Here's how the part is built. I have some questions about the finished solid (model axes, mm). A direction names the side the tool comes from. Coordinates: 2 decimals unless noted, no trailing zeros. Write each loop counter-clockwise with the first axis right and the second up, starting at its lowest first coordinate (ties: lowest second). Pieces come first, ordered by that corner, then holes.
(1) Thinking about a two-plate mould opening in X: for faces 6 (the flat face through (0, -25.5, 0)), 7 (the flat face through (0, -33.1, 0)), 8 (the cylindrical face through (37.46, -15.53, 0.99)), 9 (the flat face through (-36, -12, 0)), which applies, released by +X, released by -X, zero draft, split by the parting line, or undercut?
(2) Please list where these lines run through material, in increasing order: probe 1 along Y at (x, z) = (0, 1.15); probe 2 along X at (y, z) = (0, 2.45); probe 3 along X at (y, z) = (-32, 1).
(3) Imagine slicing it at B-B, the plane x = 0. List the corners of the cut face in (y, z) for me, plus the area to 3 significant figures.
(4) For pin 1 Ø10 at (x, y) = (30.5, -15.5) entering from -Z; pin 2 Ø1 at (x, z) = (-4.5, -1.5) entering from -Y; pin 3 Ø4 at (y, z) = (-30, 0) entering from -X, each with a flat end and sliding along its axis, tell me the tip position at first contact or that it passes through.
(5) Imagine slicing it at A-A, the plane y = 0. List the corners of the cut face in (x, z) for me.
(6) Which directions (+Z, -Z, +X, -X, +Y, -Y) give clear straight access to the entire face, cutting with the end or side of a thin tool? Please do faces 1 (the cylindrical face through (-0.1, -37.5, -2)), 2 (the flat face through (-10, -31, 0)), 3 (the flat face through (7.5, -31, 0)), 4 (the flat face through (33, -21, 1.4)), 5 (the flat face through (0, -34, -4)).
```python
from build123d import *

# Parameters (mm, degrees)
F0_R     = 40.55
F0_W     = 15
F0_H     = 5.2
F1_DEPTH = 1.4
F2_DEPTH = 3.4
F3_DEPTH = 4
F4_R     = 0.6
F5_R     = 2
F6_R     = 0.6


with BuildPart() as f1:
    # F0 (on Top) → F1 (new body)
    with BuildSketch(Plane.XY):
        Circle(F0_R)
        with BuildLine():
            ThreePointArc((-10, -37.4374478297), (-23.6015094856, 30.7332271329), (38.75, 0))
            ThreePointArc((38.75, 0), (30.7332271329, -23.6015094856), (10, -37.4374478297))
            Line((10, -37.4374478297), (10, -39))
            Line((10, -39), (-10, -39))
            Line((-10, -39), (-10, -37.4374478297))
        make_face(mode=Mode.SUBTRACT)
        with BuildLine():
            ThreePointArc((10, -37.4374478297), (30.7332271329, -23.6015094856), (38.75, 0))
            ThreePointArc((38.75, 0), (-23.6015094856, 30.7332271329), (-10, -37.4374478297))
            Line((-10, -37.4374478297), (-10, -36.142080737))
            ThreePointArc((-10, -36.142080737), (-22.7073776557, 29.8433409658), (37.5, 0))
            ThreePointArc((37.5, 0), (29.8433409658, -22.7073776557), (10, -36.142080737))
            Line((10, -36.142080737), (10, -37.4374478297))
        make_face()
        with BuildLine():
            Line((-10, -25.5), (-10, -36.142080737))
            ThreePointArc((-10, -36.142080737), (0, -37.5), (10, -36.142080737))
            Line((10, -36.142080737), (10, -25.5))
            Line((10, -25.5), (-10, -25.5))
        make_face()
        with Locations((0, -30.5)):
            Rectangle(F0_W, F0_H, mode=Mode.SUBTRACT)
        with BuildLine():
            Line((-10, -36.142080737), (-10, -37.4374478297))
            ThreePointArc((-10, -37.4374478297), (0, -38.75), (10, -37.4374478297))
            Line((10, -37.4374478297), (10, -36.142080737))
            ThreePointArc((10, -36.142080737), (0, -37.5), (-10, -36.142080737))
        make_face()
        with BuildLine():
            ThreePointArc((10, -37.4374478297), (0, -38.75), (-10, -37.4374478297))
            Line((-10, -37.4374478297), (-10, -39))
            Line((-10, -39), (10, -39))
            Line((10, -39), (10, -37.4374478297))
        make_face()
    extrude(amount=F1_DEPTH)

    # F0 (on Top) → F2 (join)
    with BuildSketch(Plane.XY):
        with BuildLine():
            ThreePointArc((10, -37.4374478297), (30.7332271329, -23.6015094856), (38.75, 0))
            ThreePointArc((38.75, 0), (-23.6015094856, 30.7332271329), (-10, -37.4374478297))
            Line((-10, -37.4374478297), (-10, -36.142080737))
            ThreePointArc((-10, -36.142080737), (-22.7073776557, 29.8433409658), (37.5, 0))
            ThreePointArc((37.5, 0), (29.8433409658, -22.7073776557), (10, -36.142080737))
            Line((10, -36.142080737), (10, -37.4374478297))
        make_face()
        with BuildLine():
            Line((-10, -36.142080737), (-10, -37.4374478297))
            ThreePointArc((-10, -37.4374478297), (0, -38.75), (10, -37.4374478297))
            Line((10, -37.4374478297), (10, -36.142080737))
            ThreePointArc((10, -36.142080737), (0, -37.5), (-10, -36.142080737))
        make_face()
        with BuildLine():
            Line((-10, -25.5), (-10, -36.142080737))
            ThreePointArc((-10, -36.142080737), (0, -37.5), (10, -36.142080737))
            Line((10, -36.142080737), (10, -25.5))
            Line((10, -25.5), (-10, -25.5))
        make_face()
        with Locations((0, -30.5)):
            Rectangle(F0_W, F0_H, mode=Mode.SUBTRACT)
    extrude(amount=F2_DEPTH)

    # F0 (on Top) → F3 (join)
    with BuildSketch(Plane.XY):
        with BuildLine():
            Line((-10, -25.5), (-10, -36.142080737))
            ThreePointArc((-10, -36.142080737), (0, -37.5), (10, -36.142080737))
            Line((10, -36.142080737), (10, -25.5))
            Line((10, -25.5), (-10, -25.5))
        make_face()
        with Locations((0, -30.5)):
            Rectangle(F0_W, F0_H, mode=Mode.SUBTRACT)
    extrude(amount=-F3_DEPTH)

    # F4
    f4_edges = [f1.edges().sort_by_distance(p)[0] for p in [
        (-40.55, 0, 0),
    ]]
    fillet(f4_edges, radius=F4_R)

    # F5
    f5_edges = [f1.edges().sort_by_distance(p)[0] for p in [
        (-10, -25.5, -0.3),
        (10, -25.5, -0.3),
        (10, -36.142081, 1.7),
        (-10, -36.142081, 1.7),
    ]]
    fillet(f5_edges, radius=F5_R)

    # F6
    f6_edges = [f1.edges().sort_by_distance(p)[0] for p in [
        (7.5, -30.5, 3.4),
        (0, -27.9, 3.4),
        (-7.5, -30.5, 3.4),
        (0, -33.1, 3.4),
        (-7.5, -30.5, -4),
        (0, -27.9, -4),
        (7.5, -30.5, -4),
        (0, -33.1, -4),
    ]]
    fillet(f6_edges, radius=F6_R)


solid = f1.part
```
Recorded:
1. face 6: undercut
1. face 7: undercut
1. face 8: split by the parting line
1. face 9: zero draft
2. probe 1: y = -40.55 to -33.1, -27.9 to -25.5, 37.5 to 40.55
2. probe 2: x = -38.75 to -37.5, 37.5 to 38.75
2. probe 3: x = -24.91 to -19.55, -10 to -7.5, 7.5 to 10, 19.55 to 24.91
3. outline: (-40.55, 0.6) arc R0.6 ccw to (-39.95, 0) - (-37.5, 0) - (-37.5, -4) - (-33.7, -4) arc R0.6 ccw to (-33.1, -3.4) - (-33.1, 2.8) arc R0.6 ccw to (-33.7, 3.4) - (-38.75, 3.4) - (-38.75, 1.4) - (-40.55, 1.4) - close; (-27.9, -3.4) arc R0.6 ccw to (-27.3, -4) - (-25.5, -4) - (-25.5, 3.4) - (-27.3, 3.4) arc R0.6 ccw to (-27.9, 2.8) - close; (37.5, 0) - (39.95, 0) arc R0.6 ccw to (40.55, 0.6) - (40.55, 1.4) - (38.75, 1.4) - (38.75, 3.4) - (37.5, 3.4) - close
3. area: 63.4 mm2
4. pin 1: stops at z = 0
4. pin 2: stops at y = -37.29
4. pin 3: stops at x = -29.26
5. outline: (-40.55, 0.6) arc R0.6 ccw to (-39.95, 0) - (-37.5, 0) - (-37.5, 3.4) - (-38.75, 3.4) - (-38.75, 1.4) - (-40.55, 1.4) - close; (37.5, 0) - (39.95, 0) arc R0.6 ccw to (40.55, 0.6) - (40.55, 1.4) - (38.75, 1.4) - (38.75, 3.4) - (37.5, 3.4) - close
6. face 1: -Z, -Y
6. face 2: -Z
6. face 3: +Z, -Z
6. face 4: +Z
6. face 5: -Z, +X, -X, +Y, -Y
